from build123d import *

# Parameters (mm, degrees)
BOX_W          = 140
BOX_H          = 20
BOX_DEPTH      = 80
BOX_ROLL_ANGLE = 12
SKETCH_W       = 140
SKETCH_H       = 95
PAD_DEPTH      = 35
SKETCH001_R    = 16.5
POCKET_DEPTH   = 34
FILLET_R       = 7
FILLET001_R    = 2
CHAMFER_SIZE   = 2
FILLET002_R    = 4


with BuildPart() as cube:
    # Box → Box (new body)
    with BuildSketch(Plane.XY):
        with Locations((70, 10)):
            Rectangle(BOX_W, BOX_H)
    extrude(amount=BOX_DEPTH)


with BuildPart() as cube_1:
    # Box roll: moved
    add(cube.part.rotate(Axis((0, 0, 0), (1, 0, 0)), BOX_ROLL_ANGLE))


with BuildPart() as cube_2:
    # Box placement: moved
    add(cube_1.part.moved(Location((-70, -59, -3))))


with BuildPart() as fillet002:
    # Sketch → Pad (new body)
    with BuildSketch(Plane.XY):
        Rectangle(SKETCH_W, SKETCH_H)
    extrude(amount=PAD_DEPTH)

    # Sketch001 → Pocket (cut)
    with BuildSketch(Plane.XY.offset(35)):
        with Locations((-45, 20.5)):
            Circle(SKETCH001_R)
        with Locations((0, 20.5)):
            Circle(SKETCH001_R)
        with Locations((45, 20.5)):
            Circle(SKETCH001_R)
        with Locations((45, -24)):
            Circle(SKETCH001_R)
        with Locations((0, -24)):
            Circle(SKETCH001_R)
        with Locations((-45, -24)):
            Circle(SKETCH001_R)
    extrude(amount=-POCKET_DEPTH, mode=Mode.SUBTRACT)

    # Fillet
    fillet_edges = [fillet002.edges().sort_by_distance(p)[0] for p in [
        (-70, -47.5, 17.5),
        (70, -47.5, 17.5),
        (70, 47.5, 17.5),
        (-70, 47.5, 17.5),
    ]]
    fillet(fillet_edges, radius=FILLET_R)

    # Fillet001
    fillet001_edges = [fillet002.edges().sort_by_distance(p)[0] for p in [
        (0, -47.5, 35),
        (-70, 0, 35),
        (0, 47.5, 35),
        (70, 0, 35),
    ]]
    fillet(fillet001_edges, radius=FILLET001_R)

    # Chamfer
    chamfer_edges = [fillet002.edges().sort_by_distance(p)[0] for p in [
        (-61.5, -24, 35),
        (-61.5, 20.5, 35),
        (-16.5, 20.5, 35),
        (-16.5, -24, 35),
        (28.5, 20.5, 35),
        (28.5, -24, 35),
    ]]
    chamfer(chamfer_edges, length=CHAMFER_SIZE)

    # Fusion: union Cube
    add(cube_2.part)

    # Fillet002
    fillet002_edges = [fillet002.edges().sort_by_distance(p)[0] for p in [
        (70, -65.851459, 77.330925),
        (-70, -65.851459, 77.330925),
        (0, -56.069983, 79.410042),
    ]]
    fillet(fillet002_edges, radius=FILLET002_R)


solid = fillet002.part
Read the model definition and answer for the solid it produces. Units are mm, in the model's axes. A direction names the side the tool comes from. Give positions to 0.01 mm unless a question says otherwise; leave off trailing zeros. Write each loop counter-clockwise with the first axis right and the second up, starting at its lowest first coordinate (ties: lowest second). Pieces come first, ordered by that corner, then holes. Notation, with made-up numbers: M 88,11 L 110,11 A16 cw 110,20 Z; hole C 17,49.25 d11. An arc over 180 degrees is marked long. One line per item, written item: value. Start each with the question number.
(1) Find section C-C (z = 30). Determine the outline of the cut face in (x, y).
(2) A tool of negligible diameter and unlimited length cuts with its end or side. For faces 4 (the flat face through (-45, 21, 1)), 5 (the flat face through (-1, 1, 35)), 6 (the flat face through (-0.92, -67.7, 76.94)), from which of +Z, -Z, +X, -X, +Y, -Y can it reach the whole face along a straight path? Write none if from no direction.
(3) Determine the mould class of faces 1 (the flat face through (45, 21, 1)), 2 (the flat face through (-1, 47.5, 16)), 3 (the cylindrical face through (68.8, -65.48, 76.24)) for opening direction X: pulls with the +X half, pulls with the -X half, needs draft (parallel to the pull), parting line crosses it, or undercut.
(4) Find section D-D (x = -21.5). Determine the outline of the cut face in (y, z), plus the area to 3 significant figures.
(5) Find section A-A (x = 0). Determine the outline of the cut face in (y, z), plus the area to 3 significant figures.
(6) Flat-ended cylindrical pins translate along their axes: pin 1 Ø1 at (x, z) = (35.5, 31.5) entering from -Y; pin 2 Ø8 at (x, y) = (-16.5, -50.5) entering from -Z; pin 3 Ø20 at (x, y) = (-45, -24) entering from -Z. Find the tip coordinate at first contact, or state that the pin passes through.
(7) Find section B-B (y = 20.5). Determine the outline of the cut face in (x, z), plus the area to 3 significant figures.
(8) Find the intervals of material crossed by line 1 (Y direction, x = 45, z = 18); line 2 (X direction, y = -24, z = 24); line 3 (X direction, y = 13.5, z = 13), in increasing order.
Results below:
1. outline: M -70,-66.01 L 70,-66.01 L 70,-45.57 L 67.83,-45.57 A7 ccw 70,-40.5 L 70,40.5 A7 ccw 63,47.5 L -63,47.5 A7 ccw -70,40.5 L -70,-40.5 A7 ccw -67.83,-45.57 L -70,-45.57 Z; hole C -45,-24 d33; hole C -45,20.5 d33; hole C 0,-24 d33; hole C 0,20.5 d33; hole C 45,-24 d33; hole C 45,20.5 d33
2. face 4: +Z
2. face 5: +Z, +X, -X, +Y
2. face 6: +Z, +X, -X, -Y
3. face 1: undercut
3. face 2: needs draft
3. face 3: pulls with the +X half
4. outline: M -75.63,75.25 L -59,-3 L -44.89,0 L 47.5,0 L 47.5,33 A2 ccw 45.5,35 L -45.5,35 A2 ccw -46.57,34.69 L -55.24,75.5 A4 ccw -59.98,78.58 Z
4. area: 4,760 mm^2
5. outline: M -75.63,75.25 L -59,-3 L -44.89,0 L 47.5,0 L 47.5,33 A2 ccw 45.5,35 L 39,35 L 37,33 L 37,1 L 4,1 L 4,33 L 2,35 L -5.5,35 L -7.5,33 L -7.5,1 L -40.18,1 L -39.44,1.16 L -40.5,6.16 L -40.5,33 L -42.5,35 L -45.5,35 A2 ccw -46.57,34.69 L -55.24,75.5 A4 ccw -59.98,78.58 Z
5. area: 2,510 mm^2
6. pin 1: stops at y = -66.44
6. pin 2: stops at z = -2.04
6. pin 3: stops at z = 0
7. outline: M -70,0 L 70,0 L 70,33 A2 ccw 68,35 L 63.5,35 L 61.5,33 L 61.5,1 L 28.5,1 L 28.5,33 L 26.5,35 L 18.5,35 L 16.5,33 L 16.5,1 L -16.5,1 L -16.5,33 L -18.5,35 L -26.5,35 L -28.5,33 L -28.5,1 L -61.5,1 L -61.5,33 L -63.5,35 L -68,35 A2 ccw -70,33 Z
7. area: 1,520 mm^2
8. line 1: y = -63.46 to -40.5, -7.5 to 4, 37 to 47.5
8. line 2: x = -70 to -61.5, -28.5 to -16.5, 16.5 to 28.5, 61.5 to 70
8. line 3: x = -70 to -59.94, -30.06 to -14.94, 14.94 to 30.06, 59.94 to 70
